```python
from build123d import *

# Parameters (mm, degrees)
BOSS_EXTRUDE1_DEPTH = 5
SKETCH7_OUTSIDE_W   = 26.516
SKETCH7_OUTSIDE_H   = 27.36
SKETCH7_OUTSIDE_R   = 7.5
CUT_EXTRUDE4_DEPTH  = 1
CUT_EXTRUDE4_TAPER  = 60
SKETCH8_OUTSIDE_W   = 26.516
SKETCH8_OUTSIDE_H   = 27.36
SKETCH8_OUTSIDE_R   = 7.5
CUT_EXTRUDE5_DEPTH  = 1
CUT_EXTRUDE5_TAPER  = 60
SKETCH9_R           = 5
CUT_EXTRUDE6_DEPTH  = 9


with BuildPart() as part:
    # Sketch1 → Boss-Extrude1 (new body)
    with BuildSketch(Plane(origin=(0, 0, 0), x_dir=(1, 0, 0), z_dir=(0, 1, 0))):
        Polygon((6.673205692, -5.519812116), (8.116900362, 3.019259596), (1.44369467, 8.539071712), (-6.673205692, 5.519812116), (-8.116900362, -3.019259596), (-1.44369467, -8.539071712), align=None)
    extrude(amount=BOSS_EXTRUDE1_DEPTH)

    # Sketch7 outside → Cut-Extrude4 (cut)
    with BuildSketch(Plane(origin=(0, 5, 0), x_dir=(1, 0, 0), z_dir=(0, 1, 0))):
        Rectangle(SKETCH7_OUTSIDE_W, SKETCH7_OUTSIDE_H)
        Circle(SKETCH7_OUTSIDE_R, mode=Mode.SUBTRACT)
    extrude(amount=-CUT_EXTRUDE4_DEPTH, taper=CUT_EXTRUDE4_TAPER, mode=Mode.SUBTRACT)

    # Sketch8 outside → Cut-Extrude5 (cut)
    with BuildSketch(Plane.XZ):
        Rectangle(SKETCH8_OUTSIDE_W, SKETCH8_OUTSIDE_H)
        Circle(SKETCH8_OUTSIDE_R, mode=Mode.SUBTRACT)
    extrude(amount=-CUT_EXTRUDE5_DEPTH, taper=CUT_EXTRUDE5_TAPER, mode=Mode.SUBTRACT)

    # Sketch9 → Cut-Extrude6 (cut)
    with BuildSketch(Plane(origin=(0, 5, 0), x_dir=(1, 0, 0), z_dir=(0, 1, 0))):
        Circle(SKETCH9_R)
    extrude(amount=-CUT_EXTRUDE6_DEPTH, mode=Mode.SUBTRACT)


solid = part.part
```
Check sheet for the modelled part. Datum: model origin and axes. Units: mm. Give positions to 0.01 mm unless a question says otherwise; leave off trailing zeros. Write each loop counter-clockwise with the first axis right and the second up, starting at its lowest first coordinate (ties: lowest second). Pieces come first, ordered by that corner, then holes.
Item 1: Gauge pin test, flat end, axial feed: pin 1 (2 mm diameter, centred on y = 1, z = 6.5, fed in from -X). Record the tip position at first contact, or that the pin passes through.
Item 2: Scan lines: L1, parallel to Z at x = 0, y = 3.6; L2, parallel to Z at x = 3.25, y = 3.2; L3, parallel to X at y = 4.6, z = 4. Record each from-to range of solid material in increasing order.
Item 3: Cross-section at A-A (y = 2.25). Enter the section's corners in (x, z).
Item 4: Cross-section at B-B (x = 0). Enter the section's corners in (y, z).
Item 5: Cross-section at C-C (z = 0). Enter the section's corners in (x, y).
Report:
1. pin 1: stops at x = -5.12
2. L1: z = -8 to -5, 5 to 8
2. L2: z = -7.04 to -3.8, 3.8 to 6.79
2. L3: x = -6.93 to -3, 3 to 6.93
3. outline: (-8.12, 3.02) - (-6.67, -5.52) - (1.44, -8.54) - (8.12, -3.02) - (6.67, 5.52) - (-1.44, 8.54) - close; hole circle Ø10 at (0, 0)
4. outline: (0, -7.5) - (0.29, -8) - (4.71, -8) - (5, -7.5) - (5, -5) - (0, -5) - close; (0, 5) - (5, 5) - (5, 7.5) - (4.71, 8) - (0.29, 8) - (0, 7.5) - close
5. outline: (-7.61, 0.06) - (-7.5, 0) - (-5, 0) - (-5, 5) - (-7.5, 5) - (-7.61, 4.94) - close; (5, 0) - (7.5, 0) - (7.61, 0.06) - (7.61, 4.94) - (7.5, 5) - (5, 5) - close
